Here's how the part is built. I have some questions about the finished solid (model axes, mm). A direction names the side the tool comes from. Give positions to 0.01 mm unless a question says otherwise; leave off trailing zeros. Write each loop counter-clockwise with the first axis right and the second up, starting at its lowest first coordinate (ties: lowest second). Pieces come first, ordered by that corner, then holes. Notation, with made-up numbers: M -34,2.5 L 18,2.5 A22 cw 18,17.5 Z; hole C 76.5,83.5 d6. An arc over 180 degrees is marked long. Answer as CSV lines item,"result". Start each with the question number.
Q1. Suppose I cut it at A-A (y = 0). Write out the boundary of the cut face in (x, z), then the cut area to 3 significant figures.
Q2. Suppose I cut it at D-D (y = -47.5). Write out the boundary of the cut face in (x, z).
Q3. Suppose I cut it at C-C (x = 53). Write out the boundary of the cut face in (y, z), then the cut area to 3 significant figures.
Q4. On a 3-axis mill with a long thin cutter (end or side, diameter ignored), from which of +Z, -Z, +X, -X, +Y, -Y can I reach the whole of each face in a straight line? I mean faces 4 (the cylindrical face through (45.35, -39.923, -20.765)), 5 (the flat face through (0, -30, -30)). Say none if no direction works.
Q5. If I drill on line 1 along Y through (x, z) = (46.5, 0); line 2 along Y through (x, z) = (17, 0); line 3 along X through (y, z) = (-48, 21), over which ranges is the centre line in solid material (lowest first)?
Q6. For pin 1 (5 mm diameter, centred on x = 46, z = 25.5, fed in from +Y); pin 2 (6 mm diameter, centred on x = 50, y = 6, fed in from +Z); pin 3 (12 mm diameter, centred on y = 23, z = -53, fed in from +X); pin 4 (3 mm diameter, centred on x = 33, y = 47.5, fed in from +Z), each with a flat end and sliding along its axis, tell me the tip position at first contact or that it passes through.
Q7. Thinking about a two-plate mould opening in Y: for faces 1 (the cylindrical face through (9.86, -42.594, 55.55)), 2 (the cylindrical face through (35.49, 37.18, 4.88)), 3 (the flat face through (20, -46, 1)), which applies, +Y half, -Y half, draft (parallel to the pull), parting line (faces both ways), or undercut?
```python
from build123d import *

# Parameters (mm, degrees)
SKETCH_1_R          = 70
EXTRUDE_1_DEPTH     = 70
SKETCH_2_R          = 37.5
CUT_EXTRUDE_1_DEPTH = 122.24355653
SKETCH_3_OUTSIDE_W  = 184
SKETCH_3_OUTSIDE_H  = 184
SKETCH_3_OUTSIDE_R  = 45
CUT_EXTRUDE_2_DEPTH = 50


with BuildPart() as part:
    # 草图1 → 凸台-拉伸1 (new body)
    with BuildSketch(Plane(origin=(0, 0, 0), x_dir=(0, 0, -1), z_dir=(1, 0, 0))):
        Circle(SKETCH_1_R)
    extrude(amount=EXTRUDE_1_DEPTH)

    # 草图2 → 切除-拉伸1 (cut, through all)
    with BuildSketch(Plane(origin=(70, 0, 0), x_dir=(0, 0, -1), z_dir=(1, 0, 0))):
        Circle(SKETCH_2_R)
    extrude(amount=-CUT_EXTRUDE_1_DEPTH, mode=Mode.SUBTRACT)

    # 草图3 outside → 切除-拉伸2 (cut)
    with BuildSketch(Plane(origin=(70, 0, 0), x_dir=(0, 0, -1), z_dir=(1, 0, 0))):
        Rectangle(SKETCH_3_OUTSIDE_W, SKETCH_3_OUTSIDE_H)
        Circle(SKETCH_3_OUTSIDE_R, mode=Mode.SUBTRACT)
    extrude(amount=-CUT_EXTRUDE_2_DEPTH, mode=Mode.SUBTRACT)


solid = part.part
```
Resolved:
1,outline,"M 0,-70 L 20,-70 L 20,-45 L 70,-45 L 70,-37.5 L 0,-37.5 Z; M 0,37.5 L 70,37.5 L 70,45 L 20,45 L 20,70 L 0,70 Z"
1,area,"2,050 mm^2"
2,outline,"M 0,-51.42 L 20,-51.42 L 20,51.42 L 0,51.42 Z"
3,outline,"C 0,0 d90; hole C 0,0 d75"
3,area,"1,940 mm^2"
4,face 4,"+X"
4,face 5,"+Z, -Z, -X, +Y, -Y"
5,line 1,"-45 to -37.5, 37.5 to 45"
5,line 2,"-70 to -37.5, 37.5 to 70"
5,line 3,"0 to 20"
6,pin 1,"y = 38.68"
6,pin 2,"z = 44.9"
6,pin 3,"x = 20"
6,pin 4,"through"
7,face 1,"parting line"
7,face 2,"undercut"
7,face 3,"draft"
